Design review of the part built by this model. Coordinates are the model's own, in mm. Coordinates: 2 decimals unless noted, no trailing zeros. Write each loop counter-clockwise with the first axis right and the second up, starting at its lowest first coordinate (ties: lowest second). Pieces come first, ordered by that corner, then holes. Notation, with made-up numbers: (16.25, 81.25) -> (57.25, 81.25) arc R8 cw to (57.25, 94.25) -> close; hole circle Ø1 at (54, 88). An arc over 180 degrees is marked (long way). One line per question, with ' | ' between items. Start each with the question number.
Q1. For P1, Ø5, axis at x = -7, z = 1, coming from the -Y side; P2, Ø1, axis at y = 1.5, z = -14, coming from the +X side; P3, Ø3, axis at x = -23.5, z = -18.5, coming from the +Y side; P4, Ø6, axis at y = 14.5, z = -2, coming from the -X side, all flat-tipped, find the tip position at first contact; note any pin that passes through.
Q2. Add section B-B on z = 0. State the section outline as (x, y) points.
Q3. Add section C-C on y = 4. State the section outline as (x, z) points.
Q4. Add section A-A on x = -60. State the section outline as (y, z) points.
Q5. Add section D-D on x = -44.5. State the section outline as (y, z) points.
Q6. Wall thickness on probe 1 along Z at (x, y) = (-60, 0.8); probe 2 along Y at (x, z) = (-13, -34.5); probe 3 along Z at (x, y) = (-16, 4): over which ranges is each line inside the solid? List them lowest first.
from build123d import *

# Parameters (mm, degrees)
SKETCH_W     = 80
SKETCH_H     = 80
SKETCH_R     = 9.5
PAD_DEPTH    = 2
PAD001_DEPTH = 2.5


with BuildPart() as part:
    # Sketch → Pad (new body)
    with BuildSketch(Plane.XZ):
        with Locations((-40, 0)):
            Rectangle(SKETCH_W, SKETCH_H)
        with Locations((-60, 0)):
            Circle(SKETCH_R, mode=Mode.SUBTRACT)
    extrude(amount=-PAD_DEPTH)

    # Sketch001 → Pad001 (join, symmetric)
    with BuildSketch(Plane.XY):
        Polygon((-26, 0), (-16, 20), (24, 20), (24, 12.55), (14, 12.55), (14, 7.45), (24, 7.45), (24, 0), align=None)
    extrude(amount=PAD001_DEPTH, both=True)


solid = part.part
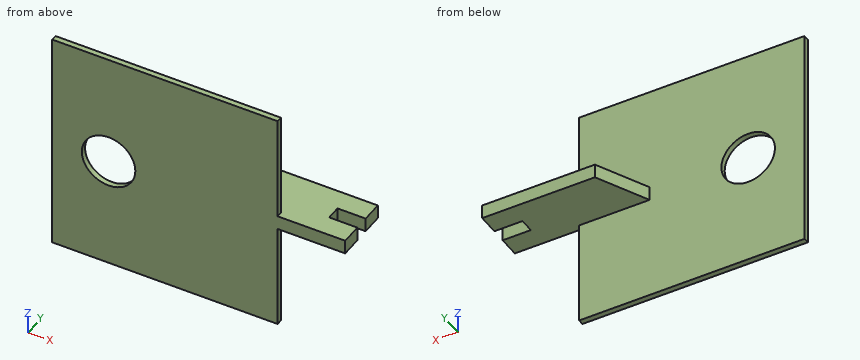
Output values:
1) P1: stops at y = 0 | P2: stops at x = 0 | P3: stops at y = 2 | P4: stops at x = -20.25
2) outline: (-80, 0) -> (-69.5, 0) -> (-69.5, 2) -> (-80, 2) -> close; (-50.5, 0) -> (24, 0) -> (24, 7.45) -> (14, 7.45) -> (14, 12.55) -> (24, 12.55) -> (24, 20) -> (-16, 20) -> (-25, 2) -> (-50.5, 2) -> close
3) outline: (-24, -2.5) -> (24, -2.5) -> (24, 2.5) -> (-24, 2.5) -> close
4) outline: (0, -40) -> (2, -40) -> (2, -9.5) -> (0, -9.5) -> close; (0, 9.5) -> (2, 9.5) -> (2, 40) -> (0, 40) -> close
5) outline: (0, -40) -> (2, -40) -> (2, 40) -> (0, 40) -> close
6) probe 1: z = -40 to -9.5, 9.5 to 40 | probe 2: y = 0 to 2 | probe 3: z = -2.5 to 2.5
